from build123d import *

# Parameters (mm, degrees)
BOSS_EXTRUDE1_DEPTH     = 20.15
CUT_EXTRUDE1_DEPTH      = 40.134529676
CUT_EXTRUDE1_DEPTH_BACK = 40.134529676
SKETCH2_R               = 3
CUT_EXTRUDE2_DEPTH      = 3.9
SKETCH5_R               = 2.3
CUT_EXTRUDE4_DEPTH      = 16.25
CUT_EXTRUDE5_START      = -15.35
SKETCH7_R               = 3.1
CUT_EXTRUDE5_DEPTH      = 23.814268799


with BuildPart() as part:
    # Sketch1 → Boss-Extrude1 (new, symmetric)
    with BuildSketch(Plane.XY):
        with BuildLine():
            Line((-27.023255814, 5), (27.023255814, 5))
            ThreePointArc((27.023255814, 5), (32.023255814, 0), (27.023255814, -5))
            Line((27.023255814, -5), (-27.023255814, -5))
            ThreePointArc((-27.023255814, -5), (-32.023255814, 0), (-27.023255814, 5))
        make_face()
    extrude(amount=BOSS_EXTRUDE1_DEPTH, both=True)

    # Sketch2 → Cut-Extrude1 (cut, two sides: drawn at the far end of the back side and taken through both)
    with BuildSketch(Plane(origin=(0, 5, 0), x_dir=(1, 0, 0), z_dir=(0, 1, 0)).offset(-CUT_EXTRUDE1_DEPTH_BACK)):
        with Locations((0, 20.15)):
            Circle(SKETCH2_R)
        with Locations((0, -20.15)):
            Circle(SKETCH2_R)
        with BuildLine():
            Line((-1.5, -14), (-1.5, 14))
            ThreePointArc((-1.5, 14), (0, 15.5), (1.5, 14))
            Line((1.5, 14), (1.5, -14))
            ThreePointArc((1.5, -14), (0, -15.5), (-1.5, -14))
        make_face()
        Polygon((27.023255814, 15.35), (38.05829872, 15.35), (38.05829872, -15.35), (27.023255814, -15.35), (3, -15.35), (3, 15.35), align=None)
        Polygon((-27.023255814, -15.35), (-38.05829872, -15.35), (-38.05829872, 15.35), (-27.023255814, 15.35), (-3, 15.35), (-3, -15.35), align=None)
    extrude(amount=CUT_EXTRUDE1_DEPTH + CUT_EXTRUDE1_DEPTH_BACK, mode=Mode.SUBTRACT)

    # Sketch4 → Cut-Extrude2 (cut)
    with BuildSketch(Plane.XY.offset(20.15)):
        with BuildLine():
            Line((25.123749299, 2.85), (12.848255814, 1.9))
            ThreePointArc((12.848255814, 1.9), (10.948255814, 0), (12.848255814, -1.9))
            Line((12.848255814, -1.9), (25.123749299, -2.85))
            ThreePointArc((25.123749299, -2.85), (30.448255814, 0), (25.123749299, 2.85))
        make_face()
        with BuildLine():
            Line((-25.123749299, 2.85), (-12.848255814, 1.9))
            ThreePointArc((-12.848255814, 1.9), (-10.948255814, 0), (-12.848255814, -1.9))
            Line((-12.848255814, -1.9), (-25.123749299, -2.85))
            ThreePointArc((-25.123749299, -2.85), (-30.448255814, 0), (-25.123749299, 2.85))
        make_face()
    extrude(amount=-CUT_EXTRUDE2_DEPTH, mode=Mode.SUBTRACT)

    # Sketch5 → Cut-Extrude4 (cut)
    with BuildSketch(Plane.XY):
        with Locations(Location((27.023255814, 0, 0), (0, 0, 180))):
            Circle(SKETCH5_R)
        with Locations(Location((-27.023255814, 0, 0), (0, 0, 180))):
            Circle(SKETCH5_R)
    extrude(amount=CUT_EXTRUDE4_DEPTH, mode=Mode.SUBTRACT)

    # Sketch7 → Cut-Extrude5 (cut, through all)
    with BuildSketch(Plane.XY.offset(CUT_EXTRUDE5_START)):
        with Locations(Location((27.023255814, 0, 0), (0, 0, 180))):
            Circle(SKETCH7_R)
        with Locations(Location((-27.023255814, 0, 0), (0, 0, 180))):
            Circle(SKETCH7_R)
    extrude(amount=-CUT_EXTRUDE5_DEPTH, mode=Mode.SUBTRACT)


solid = part.part
Geometry check sheet. Reference: the model listing, model coordinates, mm. A direction names the side the tool comes from. Give positions to 0.01 mm unless a question says otherwise; leave off trailing zeros. Order: outer loops, then holes, each group sorted by start corner. A loop starts at its lowest first (then second) coordinate and runs counter-clockwise, first axis right, second up.
1) Draft check along X on faces 1 (the cylindrical face through (-10.95, 0.04, 18.23)), 2 (the cylindrical face through (-32.022, -0.11, 17.784)), 3 (the flat face through (14.5, 2.3, 20.15)). Enter one of: released by +X, released by -X, zero draft, split by the parting line, or undercut.
Results are:
face 1: undercut
face 2: released by -X
face 3: zero draft
2) Cross-section at D-D (y = -1.25). Give the number of separate pieces and of enclosed holes in the cut face, then the cut area to 3 significant figures.
Results are:
separate pieces: 5
enclosed holes: 1
area: 469 mm2
3) Cross-section at B-B (z = 0.5). Record the boundary of the cut face in (x, y).
Results are:
outline: (-3, -5) - (-1.5, -5) - (-1.5, 5) - (-3, 5) - close; (1.5, -5) - (3, -5) - (3, 5) - (1.5, 5) - close
4) Material ranges on probe 1 along X at (y, z) = (0, 19.25); probe 2 along Z at (x, y) = (-12, 3.5); probe 3 along X at (y, z) = (-2, -4.5), recorded low to high.
Results are:
probe 1: x = -32.02 to -30.45, -10.95 to -2.86, 2.86 to 10.95, 30.45 to 32.02
probe 2: z = -20.15 to -15.35, 15.35 to 20.15
probe 3: x = -3 to -1.5, 1.5 to 3
5) Tool access check on faces 4 (the flat face through (19.07, 2.38, 18.23)), 5 (the cylindrical face through (24.066, -0.931, -17.716)), 6 (the flat face through (18, 0, -15.35)), 7 (the cylindrical face through (0, -0.1, 15.5)), 8 (the flat face through (-3, 0, 0)). Record the directions out of +Z, -Z, +X, -X, +Y, -Y that give a thin tool (end or side, any length) a straight path to the whole face; none if there is none.
Results are:
face 4: +Z
face 5: -Z
face 6: +X, +Y, -Y
face 7: +Y, -Y
face 8: -X, +Y, -Y
6) Gauge pin test, flat ends, axial feed: pin 1 (4 mm diameter, centred on x = 0.5, y = 0, fed in from -Z); pin 2 (3 mm diameter, centred on y = 1.5, z = 0.5, fed in from +X); pin 3 (5.5 mm diameter, centred on x = 16, y = -1, fed in from +Z); pin 4 (4 mm diameter, centred on y = -2, z = 12, fed in from -X). Record the tip position at first contact, or that the pin passes through.
Results are:
pin 1: stops at z = -18.49
pin 2: stops at x = 3
pin 3: stops at z = 20.15
pin 4: stops at x = -3
7) Cross-section at C-C (x = 18). Record the boundary of the cut face in (y, z).
Results are:
outline: (-5, -20.15) - (5, -20.15) - (5, -15.35) - (-5, -15.35) - close; (-5, 15.35) - (5, 15.35) - (5, 20.15) - (2.3, 20.15) - (2.3, 16.25) - (-2.3, 16.25) - (-2.3, 20.15) - (-5, 20.15) - close
8) Cross-section at A-A (x = 0). Record the boundary of the cut face in (y, z).
Results are:
outline: (-5, -17.15) - (5, -17.15) - (5, -15.5) - (-5, -15.5) - close; (-5, 15.5) - (5, 15.5) - (5, 17.15) - (-5, 17.15) - close
